Geometry check sheet. Reference: drawing and pictorial views, mm from the part's lowest x, y, z. A direction names the side the tool comes from. Give positions to 0.01 mm unless a question says otherwise; leave off trailing zeros. Write each loop counter-clockwise with the first axis right and the second up, starting at its lowest first coordinate (ties: lowest second). Pieces come first, ordered by that corner, then holes. Notation, with made-up numbers: (41, 22.5) -> (68, 22.5) arc R12 cw to (68, 44.5) -> close; hole circle Ø8 at (60, 78). An arc over 180 degrees is marked (long way). Use a Markdown table: item, result. Add a question column.
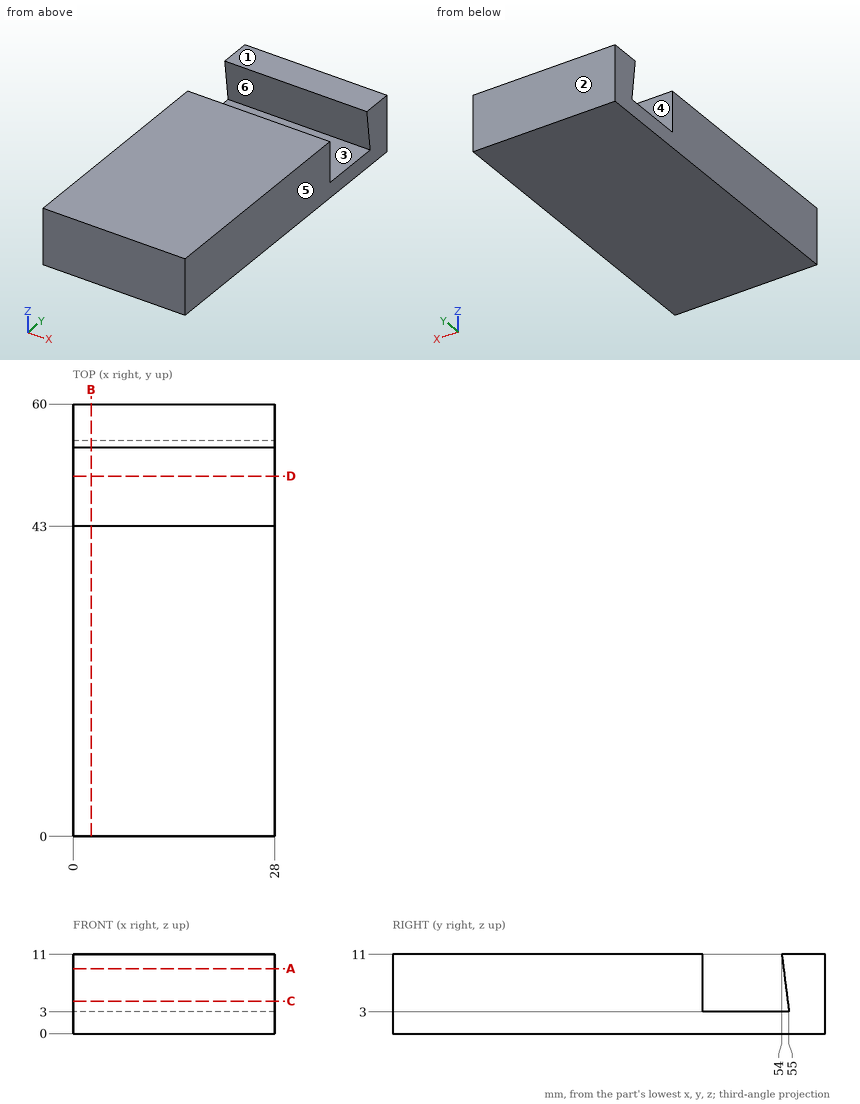
1) Sectioned sample at C-C, the plane z = 4.5. Enter the section's corners in (x, y).
2) Tool access check on the marked faces 4, 5 and 6. Record the directions out of +Z, -Z, +X, -X, +Y, -Y that give a thin tool (end or side, any length) a straight path to the whole face; none if there is none.
3) Draft check along Y on the marked faces 1, 2 and 3. Enter one of: +Y half, -Y half, draft (parallel to the pull), parting line (faces both ways), or undercut.
4) Material ranges on probe 1 along Y at (x, z) = (24, 7); probe 2 along Z at (x, y) = (10.25, 49.5); probe 3 along Y at (x, z) = (19.5, 5.5), recorded low to high. Write a range as [from, to].
5) Sectioned sample at D-D, the plane y = 50. Enter the section's corners in (x, z).
6) Sectioned sample at A-A, the plane z = 9. Enter the section's corners in (x, y), and give its area (4 significant figures).
7) Gauge pin test, flat end, axial feed: P1, Ø3.5, axis at x = 19, y = 49.5, coming from the +Z side. Record the tip position at first contact, or that the pin passes through.
8) Sectioned sample at B-B, the plane x = 2.5. Enter the section's corners in (y, z), and give its area (3 significant figures).
Check values:
| question | item | result |
|---|---|---|
| 1 | outline | (0, 0) -> (28, 0) -> (28, 43) -> (0, 43) -> close; (0, 54.81) -> (28, 54.81) -> (28, 60) -> (0, 60) -> close |
| 2 | face 4 | +Z, +X, -X |
| 2 | face 5 | +Z, -Z, +X, +Y, -Y |
| 2 | face 6 | +X, -X |
| 3 | face 1 | draft |
| 3 | face 2 | +Y half |
| 3 | face 3 | undercut |
| 4 | probe 1 | [0, 43], [54.5, 60] |
| 4 | probe 2 | [0, 3] |
| 4 | probe 3 | [0, 43], [54.69, 60] |
| 5 | outline | (0, 0) -> (28, 0) -> (28, 3) -> (0, 3) -> close |
| 6 | outline | (0, 0) -> (28, 0) -> (28, 43) -> (0, 43) -> close; (0, 54.25) -> (28, 54.25) -> (28, 60) -> (0, 60) -> close |
| 6 | area | 1,365 mm² |
| 7 | P1 | z = 3 |
| 8 | outline | (0, 0) -> (60, 0) -> (60, 11) -> (54, 11) -> (55, 3) -> (43, 3) -> (43, 11) -> (0, 11) -> close |
| 8 | area | 568 mm² |
